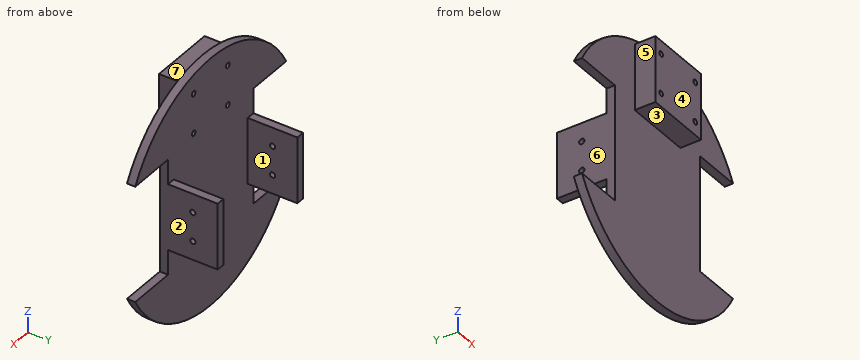
from build123d import *

# Parameters (mm, degrees)
SKETCH1_R           = 75
BOSS_EXTRUDE2_DEPTH = 5
SKETCH5_W           = 35
SKETCH5_H           = 70
CUT_EXTRUDE1_DEPTH  = 107.183802908
SKETCH6_W           = 5
SKETCH6_H           = 40
BOSS_EXTRUDE3_DEPTH = 30
SKETCH7_R           = 1.6
CUT_EXTRUDE2_DEPTH  = 136.669635512
SKETCH8_W           = 40
SKETCH8_H           = 40
BOSS_EXTRUDE5_DEPTH = 12.5
SKETCH9_R           = 1.6
CUT_EXTRUDE3_DEPTH  = 111.820801297


with BuildPart() as part:
    # Sketch1 → Boss-Extrude2 (new body)
    with BuildSketch(Plane(origin=(0, 0, 0), x_dir=(1, 0, 0), z_dir=(0, 1, 0))):
        with Locations(Location((0, 0, 0), (0, 0, 270))):
            Circle(SKETCH1_R)
    extrude(amount=BOSS_EXTRUDE2_DEPTH)

    # Sketch5 → Cut-Extrude1 (cut, through all)
    with BuildSketch(Plane(origin=(0, 5, 0), x_dir=(1, 0, 0), z_dir=(0, 1, 0))):
        with Locations((55, 0)):
            Rectangle(SKETCH5_W, SKETCH5_H)
        with Locations((-55, 0)):
            Rectangle(SKETCH5_W, SKETCH5_H)
    extrude(amount=-CUT_EXTRUDE1_DEPTH, mode=Mode.SUBTRACT)


with BuildPart() as cut_extrude1_piece_1:
    # of the separate pieces the step leaves, piece 1, a body of its own (cut_extrude1_pieces)
    add(part.part.solids().sort_by_distance((-66.332495807, 0, 35))[0])

    # Sketch6 → Boss-Extrude3 (add)
    with BuildSketch(Plane(origin=(0, 5, 0), x_dir=(1, 0, 0), z_dir=(0, 1, 0))):
        with Locations((-35, 0)):
            Rectangle(SKETCH6_W, SKETCH6_H)
    boss_extrude3 = extrude(amount=BOSS_EXTRUDE3_DEPTH)

    # Sketch7 → Cut-Extrude2 (cut, through all)
    with BuildSketch(Plane(origin=(-32.5, 0, 0), x_dir=(0, 0, -1), z_dir=(1, 0, 0))):
        with Locations((-8.75, 20)):
            Circle(SKETCH7_R)
        with Locations((8.75, 20)):
            Circle(SKETCH7_R)
    cut_extrude2 = extrude(amount=-CUT_EXTRUDE2_DEPTH, mode=Mode.SUBTRACT)

    # Mirror1: Boss-Extrude3, Cut-Extrude2 across plane
    add(boss_extrude3.mirror(Plane(origin=(0, 0, 0), x_dir=(0, 0, 1), z_dir=(1, 0, 0))))
    add(cut_extrude2.mirror(Plane(origin=(0, 0, 0), x_dir=(0, 0, 1), z_dir=(1, 0, 0))), mode=Mode.SUBTRACT)

    # Sketch8 → Boss-Extrude5 (add)
    with BuildSketch(Plane.XZ):
        with Locations((0, 50)):
            Rectangle(SKETCH8_W, SKETCH8_H)
    extrude(amount=BOSS_EXTRUDE5_DEPTH)

    # Sketch9 → Cut-Extrude3 (cut, through all)
    with BuildSketch(Plane.XZ.offset(12.5)):
        with Locations(Location((-15, 62, 0), (0, 0, 270))):
            Circle(SKETCH9_R)
        with Locations(Location((15, 62, 0), (0, 0, 270))):
            Circle(SKETCH9_R)
        with Locations(Location((-15, 38, 0), (0, 0, 270))):
            Circle(SKETCH9_R)
        with Locations(Location((15, 38, 0), (0, 0, 270))):
            Circle(SKETCH9_R)
    extrude(amount=-CUT_EXTRUDE3_DEPTH, mode=Mode.SUBTRACT)


with BuildPart() as cut_extrude1_piece_2:
    # of the separate pieces the step leaves, piece 2, a body of its own (cut_extrude1_pieces)
    add(part.part.solids().sort_by_distance((-72.5, 0, -19.20286437))[0])


with BuildPart() as cut_extrude1_piece_3:
    # of the separate pieces the step leaves, piece 3, a body of its own (cut_extrude1_pieces)
    add(part.part.solids().sort_by_distance((72.5, 0, 19.20286437))[0])


solid = cut_extrude1_piece_1.part
Could you check a few things on this model? Use its own coordinates, in mm. Face numbers are marked on the shaded views. A direction names the side the tool comes from. Give positions to 0.01 mm unless a question says otherwise; leave off trailing zeros. Write each loop counter-clockwise with the first axis right and the second up, starting at its lowest first coordinate (ties: lowest second). Pieces come first, ordered by that corner, then holes. Notation, with made-up numbers: (74, 61) - (110, 61) arc R34 ccw to (110, 99) - close; hole circle Ø2 at (-15.75, 62.25). An arc over 180 degrees is marked (long way). Use CSV: the item, a comma, the result in double quotes. Start each with the question number.
Item 1: I'm going to push flat-ended pins straight in: pin 1 (4 mm diameter, centred on x = 7, y = -4.5, fed in from -Z); pin 2 (1.9 mm diameter, centred on x = 15, z = 62, fed in from -Y) (3 decimals); pin 3 (2 mm diameter, centred on x = -44, z = -50, fed in from +Y); pin 4 (4 mm diameter, centred on y = 20, z = -8.75, fed in from +X). Where does each tip first touch, or does it pass through?
Item 2: I want a section at A-A, the plane y = 11. Please give me the cut outline in (x, z), then the cut area to 3 significant figures.
Item 3: I want a section at D-D, the plane x = -6.5. Please give me the cut outline in (y, z).
Item 4: If we mould it in two halves opening along Z, with no side actions, what happens to the marked faces 5, 6 and 7? For each: pulls with the +Z half, pulls with the -Z half, needs draft (parallel to the pull), parting line crosses it, or undercut.
Item 5: For the marked faces 1, 2, 3 and 4, which set-ups out of +Z, -Z, +X, -X, +Y, -Y let a thin tool reach every point of the face, with its end or its side?
Item 6: I want a section at C-C, the plane z = 4.5. Please give me the cut outline in (x, y), then the cut area to 3 significant figures.
Item 7: If I drill on line 1 along Z through (x, y) = (34.85, 20); line 2 along X through (y, z) = (13, 0.5); line 3 along X through (y, z) = (2, 37), over which ranges is the centre line in solid material (lowest first)?
Item 8: I want a section at B-B, the plane x = 43. Please give me the cut outline in (y, z).
Findings:
1,pin 1,"stops at z = 30"
1,pin 2,"passes through"
1,pin 3,"stops at y = 5"
1,pin 4,"stops at x = 37.5"
2,outline,"(-37.5, -20) - (-32.5, -20) - (-32.5, 20) - (-37.5, 20) - close; (32.5, -20) - (37.5, -20) - (37.5, 20) - (32.5, 20) - close"
2,area,"400 mm2"
3,outline,"(-12.5, 30) - (0, 30) - (0, -74.72) - (5, -74.72) - (5, 74.72) - (0, 74.72) - (0, 70) - (-12.5, 70) - close"
4,face 5,"needs draft"
4,face 6,"undercut"
4,face 7,"pulls with the +Z half"
5,face 1,"+Z, -Z, +Y"
5,face 2,"+X, +Y, -Y"
5,face 3,"-Z, +X, -X, -Y"
5,face 4,"+Z, -Z, +X, -X, -Y"
6,outline,"(-37.5, 0) - (37.5, 0) - (37.5, 35) - (32.5, 35) - (32.5, 5) - (-32.5, 5) - (-32.5, 35) - (-37.5, 35) - close"
6,area,"675 mm2"
7,line 1,"z = -20 to -10.35, -7.15 to 7.15, 10.35 to 20"
7,line 2,"x = -37.5 to -32.5, 32.5 to 37.5"
7,line 3,"x = -65.24 to -16.25, -13.75 to 13.75, 16.25 to 65.24"
8,outline,"(0, -61.45) - (5, -61.45) - (5, -35) - (0, -35) - close; (0, 35) - (5, 35) - (5, 61.45) - (0, 61.45) - close"
